Input: part model. Units: mm. Frame: model coordinates. Give positions to 0.01 mm unless a question says otherwise; leave off trailing zeros. Loops run counter-clockwise (first coordinate to the right, second up) from the corner with the lowest first, then second, coordinate; pieces in that order, holes last. Notation, with made-up numbers: (21.5, 41) -> (37.5, 41) arc R14 cw to (37.5, 61) -> close; hole circle Ø7 at (22.25, 13). An arc over 180 degrees is marked (long way). One line per question, with ' | ' between items.
from build123d import *

# Parameters (mm, degrees)
F0_R     = 44.45
F0_R_2   = 3.175
F1_DEPTH = 25.4


with BuildPart() as f1:
    # F0 (on Front) → F1 (new body)
    with BuildSketch(Plane.XZ):
        Circle(F0_R)
        with Locations((0, -20.32)):
            Circle(F0_R_2, mode=Mode.SUBTRACT)
        with Locations((-20.32, 0)):
            Circle(F0_R_2, mode=Mode.SUBTRACT)
        Circle(F0_R_2, mode=Mode.SUBTRACT)
        with Locations((20.32, 0)):
            Circle(F0_R_2, mode=Mode.SUBTRACT)
        with Locations((0, 20.32)):
            Circle(F0_R_2, mode=Mode.SUBTRACT)
    extrude(amount=F1_DEPTH)


solid = f1.part
1. Ray query, line 1 along Z through (x, y) = (0, -6.25) (3 decimals); line 2 along X through (y, z) = (-9.25, -2); line 3 along Z through (x, y) = (23, -14). Return the intervals inside material, ascending. Write a range as from..to.
Determined:
line 1: z = -44.45..-23.495, -17.145..-3.175, 3.175..17.145, 23.495..44.45 | line 2: x = -44.4..-22.79, -17.85..-2.47, 2.47..17.85, 22.79..44.4 | line 3: z = -38.04..-1.7, 1.7..38.04
2. Section query A-A (z = 0). Output: boundary loops of the cut face in (x, y) (3 decimals).
Determined:
outline: (-44.45, -25.4) -> (-23.495, -25.4) -> (-23.495, 0) -> (-44.45, 0) -> close; (-17.145, -25.4) -> (-3.175, -25.4) -> (-3.175, 0) -> (-17.145, 0) -> close; (3.175, -25.4) -> (17.145, -25.4) -> (17.145, 0) -> (3.175, 0) -> close; (23.495, -25.4) -> (44.45, -25.4) -> (44.45, 0) -> (23.495, 0) -> close
3. Pin query (flat end, axial travel): P1, Ø4, axis at x = 18, y = -5.5, coming from the +Z side; P2, Ø1, axis at y = -13.5, z = 34.5, coming from the +X side; P3, Ø1.5, axis at x = -12, y = -10, coming from the -Z side. Return the tip coordinate at first contact, or that it passes through.
Determined:
P1: stops at z = 41.47 | P2: stops at x = 28.63 | P3: stops at z = -43
4. Section query C-C (x = -20.32). Output: boundary loops of the cut face in (y, z) (3 decimals), then the cut area to 3 significant figures.
Determined:
outline: (-25.4, -39.534) -> (0, -39.534) -> (0, -3.175) -> (-25.4, -3.175) -> close; (-25.4, 3.175) -> (0, 3.175) -> (0, 39.534) -> (-25.4, 39.534) -> close | area: 1,850 mm2
5. Pull-direction query (X, two-part tool) for faces 1 (the flat face through (-1, -25.4, -9)), 2 (the cylindrical face through (-0.69, -12.52, -3.1)), 3 (the cylindrical face through (42.397, -12.522, 13.352)), 4 (the cylindrical face through (17.15, -12.52, 0.14)); classes: pulls with the +X half, pulls with the -X half, needs draft (parallel to the pull), parting line crosses it, or undercut.
Determined:
face 1: needs draft | face 2: undercut | face 3: parting line crosses it | face 4: undercut
6. Section query D-D (y = -7). Output: boundary loops of the cut face in (x, z) (3 decimals).
Determined:
outline: circle Ø88.9 at (0, 0); hole circle Ø6.35 at (-20.32, 0); hole circle Ø6.35 at (0, -20.32); hole circle Ø6.35 at (0, 0); hole circle Ø6.35 at (0, 20.32); hole circle Ø6.35 at (20.32, 0)
7. Section query B-B (x = 0). Output: boundary loops of the cut face in (y, z) (3 decimals), then the cut area to 3 significant figures.
Determined:
outline: (-25.4, -44.45) -> (0, -44.45) -> (0, -23.495) -> (-25.4, -23.495) -> close; (-25.4, -17.145) -> (0, -17.145) -> (0, -3.175) -> (-25.4, -3.175) -> close; (-25.4, 3.175) -> (0, 3.175) -> (0, 17.145) -> (-25.4, 17.145) -> close; (-25.4, 23.495) -> (0, 23.495) -> (0, 44.45) -> (-25.4, 44.45) -> close | area: 1,770 mm2
